Geometry check sheet. Reference: drawing and pictorial views, mm from the part's lowest x, y, z. A direction names the side the tool comes from. Coordinates: 2 decimals unless noted, no trailing zeros. Loops run counter-clockwise (first coordinate to the right, second up) from the corner with the lowest first, then second, coordinate; pieces in that order, holes last.
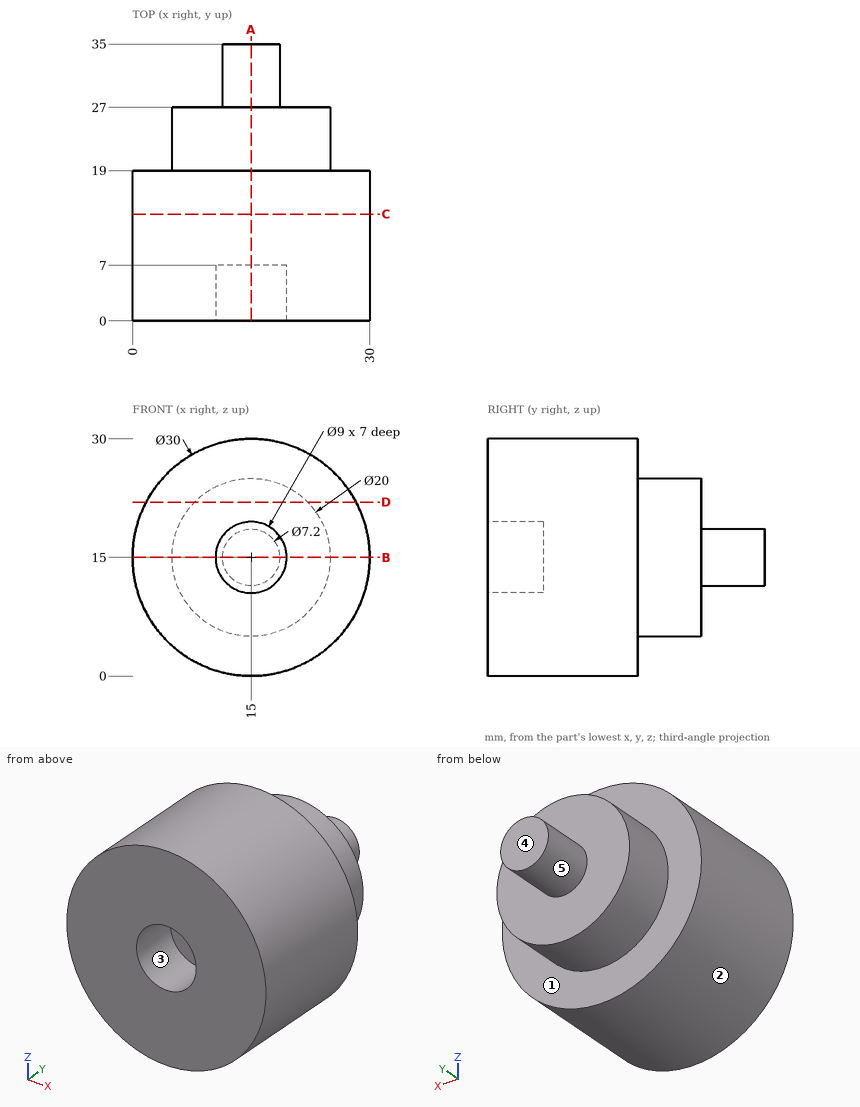
1) Mould release check, pull along X, two halves, no side actions. Record for the marked faces 1, 2 and 3: +X half, -X half, draft (parallel to the pull), parting line (faces both ways), or undercut.
Data:
face 1: draft
face 2: parting line
face 3: undercut
2) Depth check by flat-ended pin: pin 1 (2 mm diameter, centred on x = 25, y = 19, fed in from +Z); pin 2 (8 mm diameter, centred on x = 14.5, y = 22.5, fed in from -Z); pin 3 (5 mm diameter, centred on x = 23, z = 14.5, fed in from +Y); pin 4 (4 mm diameter, centred on x = 19, y = 15.5, fed in from +Z). Enter the tip coordinate at first touch or a pass-through.
Data:
pin 1: stops at z = 27
pin 2: stops at z = 0
pin 3: stops at y = 27
pin 4: stops at z = 29.87
3) Material ranges on probe 1 along Z at (x, y) = (15, 4.75); probe 2 along Y at (x, z) = (9.25, 27.25); probe 3 along Y at (x, z) = (22.25, 21.75), recorded low to high.
Data:
probe 1: z = 0 to 10.5, 19.5 to 30
probe 2: y = 0 to 19
probe 3: y = 0 to 27
4) Access from +Z, -Z, +X, -X, +Y, -Y to the whole of each face (thin tool, end or side, straight path). Record for the marked faces 4 and 5.
Data:
face 4: +Z, -Z, +X, -X, +Y
face 5: +Y
5) Section check A-A on x = 15. Record the cut outline in (y, z), and give its area (3 significant figures).
Data:
outline: (0, 0) - (19, 0) - (19, 5) - (27, 5) - (27, 11.4) - (35, 11.4) - (35, 18.6) - (27, 18.6) - (27, 25) - (19, 25) - (19, 30) - (0, 30) - (0, 19.5) - (7, 19.5) - (7, 10.5) - (0, 10.5) - close
area: 725 mm2
6) Section check B-B on z = 15. Record the cut outline in (x, y).
Data:
outline: (0, 0) - (10.5, 0) - (10.5, 7) - (19.5, 7) - (19.5, 0) - (30, 0) - (30, 19) - (25, 19) - (25, 27) - (18.6, 27) - (18.6, 35) - (11.4, 35) - (11.4, 27) - (5, 27) - (5, 19) - (0, 19) - close
7) Section check C-C on y = 13.5. Record the cut outline in (x, z).
Data:
outline: circle Ø30 at (15, 15)
8) Section check D-D on z = 22. Record the cut outline in (x, y), and give its area (3 significant figures).
Data:
outline: (1.73, 0) - (28.27, 0) - (28.27, 19) - (22.14, 19) - (22.14, 27) - (7.86, 27) - (7.86, 19) - (1.73, 19) - close
area: 618 mm2
